Geometry: final body of the model. Coordinates: model frame, mm. A direction names the side the tool comes from. Round coordinates to 2 decimals unless told otherwise and drop trailing zeros. Write each loop counter-clockwise with the first axis right and the second up, starting at its lowest first coordinate (ties: lowest second). Pieces come first, ordered by that corner, then holes. Notation, with made-up numbers: (-35.5, -28) -> (-7.5, -28) arc R23 ccw to (-7.5, 11) -> close; hole circle Ø4 at (70.5, 25.25). An arc over 180 degrees is marked (long way). Use one line per item in the form item = value. Start each with the question number.
1. Cut plane B-B, the plane y = 10.75. Return the cut outline in (x, z) (3 decimals).
2. Cut plane A-A, the plane x = -4.5. Return the cut outline in (y, z), plus the area to 3 significant figures.
3. Cut plane C-C, the plane y = 16.25. Return the cut outline in (x, z) (3 decimals).
4. Line query: L1, parallel to Y at x = -9.5, z = 0; L2, parallel to Y at x = 0.5, z = -8.4 (3 decimals); L3, parallel to Z at x = -3, y = 4.75. Output: solid intervals per line, ascending.
5. Pin query (flat end, axial travel): pin 1 Ø3 at (x, y) = (0.5, 13) entering from +Z; pin 2 Ø2.5 at (y, z) = (7.5, -9) entering from -X; pin 3 Ø4 at (x, y) = (-13.5, 11) entering from -Z. Return the tip coordinate at first contact, or that it passes through.
6. Cut plane D-D, the plane x = 0.5. Return the cut outline in (y, z) (3 decimals).
7. Reachability of faces 5 (the face through (-13, 15, 1.5)), 6 (the face through (-4.773, 11.082, -6.451)), 7 (the face through (-19.68, 15.04, 11.72)), 8 (the face through (-22.625, 0.507, 3.185)) from +Z, -Z, +X, -X, +Y, -Y: full face, straight path, thin tool, end or side. Return the list, or none.
8. Draft query along Z for faces 1 (the face through (-15.762, 2.958, 6.794)), 2 (the face through (-25, 9, 7)), 3 (the face through (-11.986, 9.112, -2.988)), 4 (the face through (-6, 0, 1)). Return one class per face: pulls with the +Z half, pulls with the -Z half, needs draft (parallel to the pull), parting line crosses it, or undercut.
```python
from build123d import *

# Parameters (mm, degrees)
SKETCH_1_R             = 2.51
SKETCH_1_R_2           = 2.525
EXTRUDE_1_DEPTH        = 18
SKETCH_11_R            = 3.75
CUT_EXTRUDE_5_DEPTH    = 6
FILLET_1_R             = 8
SKETCH_12_R            = 2
CUT_EXTRUDE_6_DEPTH    = 7
CHAMFER_1_SIZE         = 1
CUT_EXTRUDE_8_DEPTH    = 6
SKETCH_18_R            = 1.015
CUT_EXTRUDE_10_DEPTH   = 4
CUT_EXTRUDE_11_DEPTH   = 16
HOLE_WIZARD_M5_1_D     = 4.2
HOLE_WIZARD_M5_1_DEPTH = 7


with BuildPart() as part:
    # 草图1 → 凸台-拉伸1 (new body)
    with BuildSketch(Plane(origin=(0, 0, 0), x_dir=(1, 0, 0), z_dir=(0, 1, 0))):
        with BuildLine():
            Line((-21.381110788, -1.929110154), (-10.5, 2.031290289))
            Line((-10.5, 2.031290289), (-10.5, 10))
            Line((-10.5, 10), (5.5, 10))
            Line((5.5, 10), (5.5, 0))
            ThreePointArc((5.5, 0), (4.505336244, -3.1546704), (1.881110788, -5.168309414))
            Line((1.881110788, -5.168309414), (-17.618889212, -12.265728983))
            ThreePointArc((-17.618889212, -12.265728983), (-24.668309414, -8.978530356), (-21.381110788, -1.929110154))
        make_face()
        with Locations(Location((-19.5, -7.097419568, 0), (0, 0, 270))):
            Circle(SKETCH_1_R, mode=Mode.SUBTRACT)
        with Locations(Location((-2.585532826, -0.941056988, 0), (0, 0, 270))):
            Circle(SKETCH_1_R_2, mode=Mode.SUBTRACT)
    extrude(amount=EXTRUDE_1_DEPTH)

    # 草图11 → 切除-拉伸5 (cut)
    with BuildSketch(Plane(origin=(0, 18, 0), x_dir=(1, 0, 0), z_dir=(0, 1, 0))):
        with Locations(Location((-19.5, -7.097419568, 0), (0, 0, 270))):
            Circle(SKETCH_11_R)
    cut_extrude_5 = extrude(amount=-CUT_EXTRUDE_5_DEPTH, mode=Mode.SUBTRACT)

    # 圆角1
    fillet_1_edges = [part.edges().sort_by_distance(p)[0] for p in [
        (-10.5, 9, -2.031290289),
    ]]
    fillet(fillet_1_edges, radius=FILLET_1_R)

    # 草图12 → 切除-拉伸6 (cut)
    with BuildSketch(Plane(origin=(0, 0, -10), x_dir=(-1, 0, 0), z_dir=(0, 0, -1))):
        with Locations((4.5, 9)):
            Circle(SKETCH_12_R)
    extrude(amount=-CUT_EXTRUDE_6_DEPTH, mode=Mode.SUBTRACT)

    # 倒角1
    chamfer_1_edges = [part.edges().sort_by_distance(p)[0] for p in [
        (-24.668309414, 0, 8.978530356),
        (4.505336244, 18, 3.1546704),
        (5.5, 18, -5),
        (-10.5, 18, -8.816475297),
        (-18.572474821, 0, 0.906850263),
        (-18.572474821, 18, 0.906850263),
        (-11.946783646, 0, -3.044339104),
        (-11.946783646, 18, -3.044339104),
        (-24.668309414, 18, 8.978530356),
        (-10.5, 0, -8.816475297),
        (5.5, 0, -5),
        (-7.868889212, 18, 8.717019198),
        (4.505336244, 0, 3.1546704),
        (-7.868889212, 0, 8.717019198),
    ]]
    chamfer(chamfer_1_edges, length=CHAMFER_1_SIZE)

    # 草图15 → 切除-拉伸8 (cut)
    with BuildSketch(Plane(origin=(0, 18, 0), x_dir=(1, 0, 0), z_dir=(0, 1, 0))):
        with BuildLine():
            Line((-20.782575537, -3.57357224), (-28.300116504, -6.309733387))
            Line((-28.300116504, -6.309733387), (-24.879915071, -15.706659595))
            Line((-24.879915071, -15.706659595), (-19.006836191, -13.569033699))
            Line((-19.006836191, -13.569033699), (-20.0101096, -10.81256266))
            ThreePointArc((-20.0101096, -10.81256266), (-23.228830323, -7.495319585), (-20.782575537, -3.57357224))
        make_face()
    cut_extrude_8 = extrude(amount=-CUT_EXTRUDE_8_DEPTH, mode=Mode.SUBTRACT)

    # 草图18 → 切除-拉伸10 (cut)
    with BuildSketch(Plane(origin=(0, 0, -10), x_dir=(-1, 0, 0), z_dir=(0, 0, -1))):
        with Locations((-0.5, 13)):
            Circle(SKETCH_18_R)
        with Locations(Location((-0.5, 5, 0), (0, 0, 180))):
            Circle(SKETCH_18_R)
    extrude(amount=-CUT_EXTRUDE_10_DEPTH, mode=Mode.SUBTRACT)

    # 草图19 → 切除-拉伸11 (cut)
    with BuildSketch(Plane(origin=(-21.144462086, 0, 7.695954819), x_dir=(0.3420201433256672, 0, 0.939692620785909), z_dir=(-0.9396926207859089, 0, 0.34202014332566716))):
        with BuildLine():
            Line((-3.25, 12), (-2.85, 12))
            ThreePointArc((-2.85, 12), (-2.496446609, 12.146446609), (-2.35, 12.5))
            Line((-2.35, 12.5), (-2.35, 14.5))
            ThreePointArc((-2.35, 14.5), (-2.496446609, 14.853553391), (-2.85, 15))
            Line((-2.85, 15), (-3.25, 15))
            ThreePointArc((-3.25, 15), (-3.603553391, 14.853553391), (-3.75, 14.5))
            Line((-3.75, 14.5), (-3.75, 12.5))
            ThreePointArc((-3.75, 12.5), (-3.603553391, 12.146446609), (-3.25, 12))
        make_face()
    cut_extrude_11 = extrude(amount=-CUT_EXTRUDE_11_DEPTH, mode=Mode.SUBTRACT)

    # 镜向3: 切除-拉伸5, 切除-拉伸8, 切除-拉伸11 across plane
    add(cut_extrude_5.mirror(Plane(origin=(0, 9, 0), x_dir=(0, 0, 1), z_dir=(0, -1, 0))), mode=Mode.SUBTRACT)
    add(cut_extrude_8.mirror(Plane(origin=(0, 9, 0), x_dir=(0, 0, 1), z_dir=(0, -1, 0))), mode=Mode.SUBTRACT)
    add(cut_extrude_11.mirror(Plane(origin=(0, 9, 0), x_dir=(0, 0, 1), z_dir=(0, -1, 0))), mode=Mode.SUBTRACT)

    # M5 螺纹孔1
    with Locations(Plane(origin=(0, 0, -10), x_dir=(-1, 0, 0), z_dir=(0, 0, -1))):
        with Locations((4.5, 9)):
            Hole(HOLE_WIZARD_M5_1_D / 2, depth=HOLE_WIZARD_M5_1_DEPTH)


solid = part.part
```
Outcome:
q1.outline = (-21.381, 1.929) -> (-15.764, -0.115) arc R8 cw to (-10.5, -7.633) -> (-10.5, -10) -> (-5.661, -10) -> (-5.661, -3) -> (-3.339, -3) -> (-3.339, -10) -> (5.5, -10) -> (5.5, 0) arc R5.5 ccw to (1.881, 5.168) -> (-17.619, 12.266) arc R5.5 ccw to start; hole circle Ø5.02 at (-19.5, 7.097); hole circle Ø5.05 at (-2.586, 0.941)
q2.outline = (0, -10) -> (6.9, -10) -> (6.9, -3) -> (11.1, -3) -> (11.1, -10) -> (18, -10) -> (18, -0.71) -> (0, -0.71) -> close; (0, 2.59) -> (18, 2.59) -> (18, 6.43) -> (17, 7.49) -> (1, 7.49) -> (0, 6.43) -> close
q2.area = 225 mm^2
q3.outline = (-24.563, 4.95) arc R5.5 ccw to (-21.381, 1.929) -> (-15.764, -0.115) arc R8 cw to (-10.5, -7.633) -> (-10.5, -10) -> (5.5, -10) -> (5.5, 0) arc R5.5 ccw to (1.881, 5.168) -> (-17.619, 12.266) arc R5.5 ccw to (-19.361, 12.596) -> (-20.01, 10.813) arc R3.75 cw (long way) to (-20.783, 3.574) -> close; hole circle Ø5.05 at (-2.586, 0.941)
q4.L1 = 0 to 3, 6 to 12, 15 to 18
q4.L2 = 0 to 3.985, 6.015 to 11.985, 14.015 to 18
q4.L3 = -10 to -1.55, 3.43 to 6.94
q5.pin_1 = 6.22
q5.pin_2 = -10.5
q5.pin_3 = -3.76
q6.outline = (0, -10) -> (3.985, -10) -> (3.985, -6) -> (6.015, -6) -> (6.015, -10) -> (11.985, -10) -> (11.985, -6) -> (14.015, -6) -> (14.015, -10) -> (18, -10) -> (18, 4.607) -> (17, 5.671) -> (1, 5.671) -> (0, 4.607) -> close
q7.face_5 = none
q7.face_6 = -Z
q7.face_7 = +Z, -X, +Y
q7.face_8 = -Z, -X, -Y
q8.face_1 = undercut
q8.face_2 = parting line crosses it
q8.face_3 = pulls with the -Z half
q8.face_4 = needs draft
